from build123d import *

# Parameters (mm, degrees)
SKETCH1_R           = 1.37499852
BOSS_EXTRUDE1_DEPTH = 3.048
SKETCH2_R           = 1.25
SKETCH2_W           = 6.7
SKETCH2_H           = 22.7542
SKETCH2_W_2         = 0.762
CUT_EXTRUDE1_DEPTH  = 4.048


with BuildPart() as part:
    # Sketch1 → Boss-Extrude1 (new body)
    with BuildSketch(Plane.XY):
        with BuildLine():
            Line((0.41036367, 15.02963974), (60.10036367, 15.02963974))
            ThreePointArc((60.10036367, 15.02963974), (61.896414894, 14.285690964), (62.64036367, 12.48963974))
            Line((62.64036367, 12.48963974), (62.64036367, -38.4396361))
            ThreePointArc((62.64036367, -38.4396361), (61.896414894, -40.235687324), (60.10036367, -40.9796361))
            Line((60.10036367, -40.9796361), (0.41036367, -40.9796361))
            ThreePointArc((0.41036367, -40.9796361), (-1.385687554, -40.235687324), (-2.12963633, -38.4396361))
            Line((-2.12963633, -38.4396361), (-2.12963633, 12.48963974))
            ThreePointArc((-2.12963633, 12.48963974), (-1.385687554, 14.285690964), (0.41036367, 15.02963974))
        make_face()
        with Locations((1.37500106, 11.52500108)):
            Circle(SKETCH1_R, mode=Mode.SUBTRACT)
        with Locations((59.3750019, 11.52500108)):
            Circle(SKETCH1_R, mode=Mode.SUBTRACT)
        with Locations((59.3750019, -37.47499998)):
            Circle(SKETCH1_R, mode=Mode.SUBTRACT)
        with Locations((1.37500106, -37.47499998)):
            Circle(SKETCH1_R, mode=Mode.SUBTRACT)
    extrude(amount=-BOSS_EXTRUDE1_DEPTH)

    # Sketch2 → Cut-Extrude1 (cut, through all)
    with BuildSketch(Plane.XY):
        with Locations((38.25636367, -2.00169818)):
            Circle(SKETCH2_R)
        with Locations((50.77996367, -2.00169818)):
            Circle(SKETCH2_R)
        with Locations((50.77996367, -23.57459818)):
            Circle(SKETCH2_R)
        with Locations((38.25636367, -23.57459818)):
            Circle(SKETCH2_R)
        with Locations((32.15146367, -12.97499818)):
            Rectangle(SKETCH2_W, SKETCH2_H)
        with Locations((23.34046367, -12.97499818)):
            Rectangle(SKETCH2_W_2, SKETCH2_H)
    extrude(amount=-CUT_EXTRUDE1_DEPTH, mode=Mode.SUBTRACT)


solid = part.part
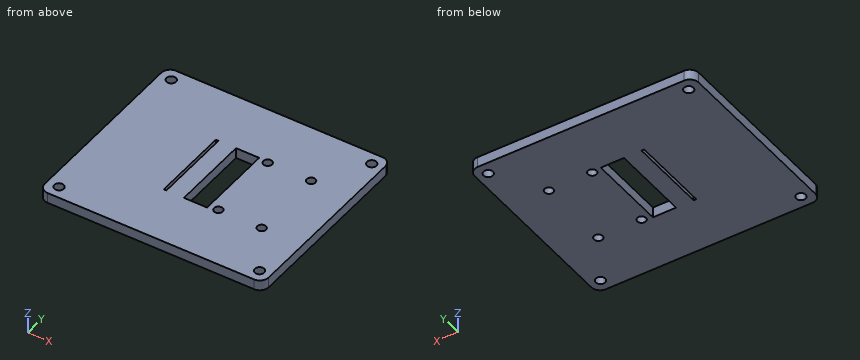
Design review of the part built by this model. Coordinates are the model's own, in mm. Coordinates: 2 decimals unless noted, no trailing zeros. Order: outer loops, then holes, each group sorted by start corner. A loop starts at its lowest first (then second) coordinate and runs counter-clockwise, first axis right, second up. Notation, with made-up numbers: (3.25, 47.25) -> (42.25, 47.25) arc R25 cw to (42.25, 69.25) -> close; hole circle Ø8 at (-36, 11.25). An arc over 180 degrees is marked (long way). One line per item, written item: value.
1) We need section A-A, the plane y = -11. Give the boundary of the cut face in (x, z).
Output values:
outline: (-2.13, -3.05) -> (22.96, -3.05) -> (22.96, 0) -> (-2.13, 0) -> close; (23.72, -3.05) -> (28.8, -3.05) -> (28.8, 0) -> (23.72, 0) -> close; (35.5, -3.05) -> (62.64, -3.05) -> (62.64, 0) -> (35.5, 0) -> close
2) We need section B-B, the plane z = -2.55. Count the separate pieces of the cut face and the enclosed holes in it, then the cut area to 3 significant figures.
Output values:
separate pieces: 1
enclosed holes: 10
area: 3,410 mm2
3) To check wall thickness, follow probe 1 along X at (y, z) = (-11, -0.85); probe 2 along X at (y, z) = (-24.5, -0.7); probe 3 along Y at (x, z) = (59, -1.9). State the ranges of each line that lie inside material, in increasing order. Write a range as [from, to].
Output values:
probe 1: x = [-2.13, 22.96], [23.72, 28.8], [35.5, 62.64]
probe 2: x = [-2.13, 37.42], [39.1, 49.94], [51.62, 62.64]
probe 3: y = [-40.98, -38.8], [-36.15, 10.2], [12.85, 15.03]
